Verification items for this drawing (mm, ordinates from the low corner). A direction names the side the tool comes from. Round coordinates to 2 decimals unless told otherwise and drop trailing zeros. Loops run counter-clockwise (first coordinate to the right, second up) from the corner with the lowest first, then second, coordinate; pieces in that order, holes last. Notation, with made-up numbers: M 55.25,-20.5 L 108.25,-20.5 A25 cw 108.25,-5.5 Z; hole C 34,-1.5 d1. An arc over 180 degrees is marked long. Answer in a Markdown table with one row per item. Add a question column.
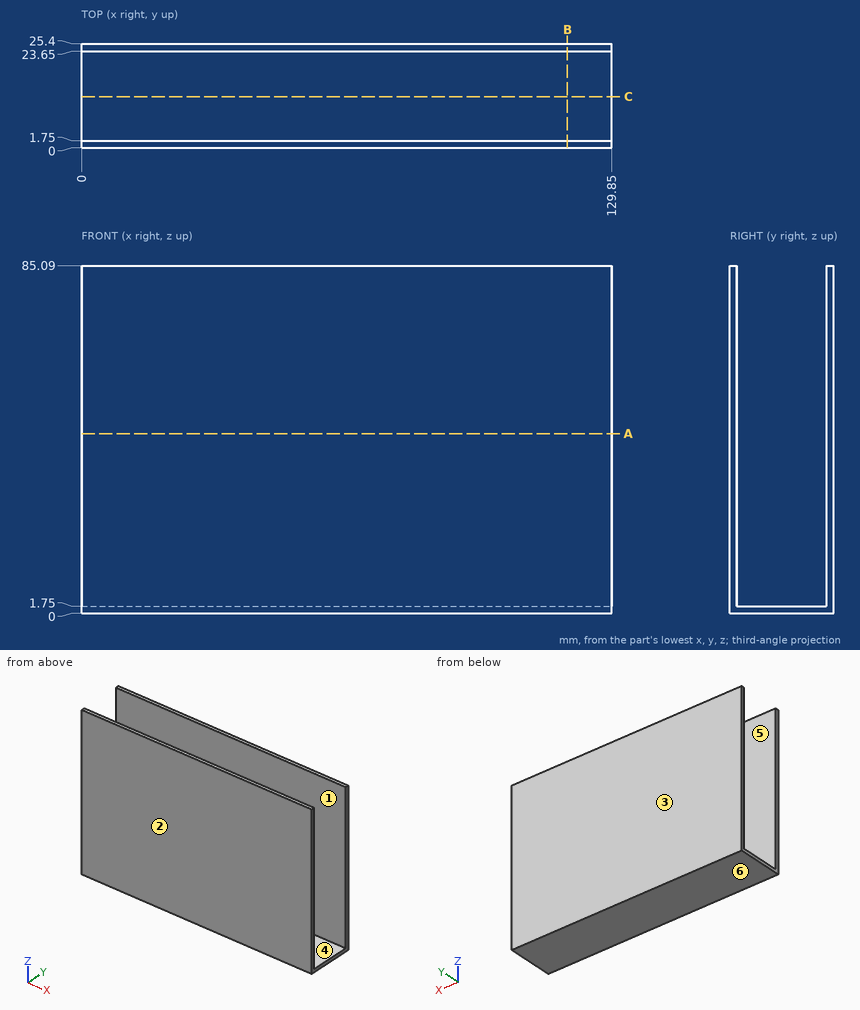
1) Cross-section at B-B, the plane x = 119. Record the boundary of the cut face in (y, z).
2) Cross-section at A-A, the plane z = 44. Record the boundary of the cut face in (x, y), plus the area to 3 significant figures.
3) Thickness scan on L1, parallel to Y at x = 21, z = 33.5; L2, parallel to Z at x = 38, y = 16. Record the ranges inside material, lowest first. Write a range as [from, to].
4) Go/stop test with a flat-tipped pin: pin 1 (1 mm diameter, centred on x = 105, y = 11, fed in from +Z). Record where the tip stops, or that it passes through.
5) Draft check along Y on the marked faces 3, 4, 5 and 6. Enter one of: +Y half, -Y half, draft (parallel to the pull), parting line (faces both ways), or undercut.
6) Cross-section at C-C, the plane y = 12.5. Record the boundary of the cut face in (x, z).
7) Set-up check for the marked faces 1 and 2: record each of +Z, -Z, +X, -X, +Y, -Y from which the full face is reachable in a straight line by a thin tool's end or side.
Worked answers:
| question | item | result |
|---|---|---|
| 1 | outline | M 0,0 L 25.4,0 L 25.4,85.09 L 23.65,85.09 L 23.65,1.75 L 1.75,1.75 L 1.75,85.09 L 0,85.09 Z |
| 2 | outline | M 0,0 L 129.85,0 L 129.85,1.75 L 0,1.75 Z; M 0,23.65 L 129.85,23.65 L 129.85,25.4 L 0,25.4 Z |
| 2 | area | 454 mm2 |
| 3 | L1 | y = [0, 1.75], [23.65, 25.4] |
| 3 | L2 | z = [0, 1.75] |
| 4 | pin 1 | stops at z = 1.75 |
| 5 | face 3 | +Y half |
| 5 | face 4 | undercut |
| 5 | face 5 | undercut |
| 5 | face 6 | draft |
| 6 | outline | M 0,0 L 129.85,0 L 129.85,1.75 L 0,1.75 Z |
| 7 | face 1 | +Z, +X, -X |
| 7 | face 2 | +Z, -Z, +X, -X, -Y |
